from build123d import *

# Parameters (mm, degrees)
SKETCH_1_W          = 4.5
SKETCH_1_H          = 8
EXTRUDE_1_DEPTH     = 30
SKETCH_4_R          = 2.5
CUT_EXTRUDE_2_DEPTH = 32.372758884
SKETCH_7_R          = 3.5
CUT_EXTRUDE_4_DEPTH = 0.5
FILLET_1_R          = 1


with BuildPart() as part:
    # 草图1 → 凸台-拉伸1 (new body)
    with BuildSketch(Plane.XY):
        with Locations((2.25, 4)):
            Rectangle(SKETCH_1_W, SKETCH_1_H)
    extrude(amount=EXTRUDE_1_DEPTH)

    # 草图4 → 切除-拉伸2 (cut, through all)
    with BuildSketch(Plane(origin=(4.5, 0, 0), x_dir=(0, 0, -1), z_dir=(1, 0, 0))):
        with Locations((-5, 4)):
            Circle(SKETCH_4_R)
        with Locations((-22, 4)):
            Circle(SKETCH_4_R)
    extrude(amount=-CUT_EXTRUDE_2_DEPTH, mode=Mode.SUBTRACT)

    # 草图7 → 切除-拉伸4 (cut)
    with BuildSketch(Plane.ZY):
        with Locations((5, 4)):
            Circle(SKETCH_7_R)
        with Locations((22, 4)):
            Circle(SKETCH_7_R)
    extrude(amount=-CUT_EXTRUDE_4_DEPTH, mode=Mode.SUBTRACT)

    # 圆角1
    # the kernel refuses this fillet: 1 mm, written as the material it takes off along each edge
    with BuildSketch(Plane(origin=(3.5, 7, 29), x_dir=(1, 0, 0), z_dir=(0, 1, 0))) as fillet_1_piece_1_section:
        Polygon((0, 0), (FILLET_1_R, 0), (FILLET_1_R, -FILLET_1_R), (0, -FILLET_1_R), align=None)
    fillet_1_piece_1 = extrude(amount=FILLET_1_R, mode=Mode.PRIVATE)
    fillet_1_piece_1 = fillet_1_piece_1 - Plane(origin=(3.5, 7, 29), x_dir=(-0.7071067811865475, 0, -0.7071067811865475), z_dir=(0, 1, 0)) * Sphere(FILLET_1_R, mode=Mode.PRIVATE)
    add(fillet_1_piece_1, mode=Mode.SUBTRACT)
    with BuildSketch(Plane(origin=(3.5, 1, 29), x_dir=(0, 0, 1), z_dir=(1, 0, 0))) as fillet_1_piece_2_section:
        Polygon((0, 0), (FILLET_1_R, 0), (FILLET_1_R, FILLET_1_R), (0, FILLET_1_R), align=None)
    fillet_1_piece_2 = extrude(amount=FILLET_1_R, mode=Mode.PRIVATE)
    fillet_1_piece_2 = fillet_1_piece_2 - Plane(origin=(3.5, 1, 29), x_dir=(0, 0.7071067811865475, -0.7071067811865475), z_dir=(1, 0, 0)) * Sphere(FILLET_1_R, mode=Mode.PRIVATE)
    add(fillet_1_piece_2, mode=Mode.SUBTRACT)
    with BuildSketch(Plane(origin=(1, 7, 29), x_dir=(-1, 0, 0), z_dir=(0, 1, 0))) as fillet_1_piece_3_section:
        Polygon((0, 0), (FILLET_1_R, 0), (FILLET_1_R, FILLET_1_R), (0, FILLET_1_R), align=None)
    fillet_1_piece_3 = extrude(amount=FILLET_1_R, mode=Mode.PRIVATE)
    fillet_1_piece_3 = fillet_1_piece_3 - Plane(origin=(1, 7, 29), x_dir=(0.7071067811865475, 0, -0.7071067811865475), z_dir=(0, 1, 0)) * Sphere(FILLET_1_R, mode=Mode.PRIVATE)
    add(fillet_1_piece_3, mode=Mode.SUBTRACT)
    with BuildSketch(Plane(origin=(1, 1, 29), x_dir=(0, 0, 1), z_dir=(-1, 0, 0))) as fillet_1_piece_4_section:
        Polygon((0, 0), (FILLET_1_R, 0), (FILLET_1_R, -FILLET_1_R), (0, -FILLET_1_R), align=None)
    fillet_1_piece_4 = extrude(amount=FILLET_1_R, mode=Mode.PRIVATE)
    fillet_1_piece_4 = fillet_1_piece_4 - Plane(origin=(1, 1, 29), x_dir=(0, 0.7071067811865475, -0.7071067811865475), z_dir=(-1, 0, 0)) * Sphere(FILLET_1_R, mode=Mode.PRIVATE)
    add(fillet_1_piece_4, mode=Mode.SUBTRACT)
    with BuildSketch(Plane(origin=(1, 7, 1), x_dir=(-1, 0, 0), z_dir=(0, 1, 0))) as fillet_1_piece_5_section:
        Polygon((0, 0), (FILLET_1_R, 0), (FILLET_1_R, -FILLET_1_R), (0, -FILLET_1_R), align=None)
    fillet_1_piece_5 = extrude(amount=FILLET_1_R, mode=Mode.PRIVATE)
    fillet_1_piece_5 = fillet_1_piece_5 - Plane(origin=(1, 7, 1), x_dir=(0.7071067811865475, 0, 0.7071067811865475), z_dir=(0, 1, 0)) * Sphere(FILLET_1_R, mode=Mode.PRIVATE)
    add(fillet_1_piece_5, mode=Mode.SUBTRACT)
    with BuildSketch(Plane(origin=(3.5, 7, 1), x_dir=(1, 0, 0), z_dir=(0, 1, 0))) as fillet_1_piece_6_section:
        Polygon((0, 0), (FILLET_1_R, 0), (FILLET_1_R, FILLET_1_R), (0, FILLET_1_R), align=None)
    fillet_1_piece_6 = extrude(amount=FILLET_1_R, mode=Mode.PRIVATE)
    fillet_1_piece_6 = fillet_1_piece_6 - Plane(origin=(3.5, 7, 1), x_dir=(-0.7071067811865475, 0, 0.7071067811865475), z_dir=(0, 1, 0)) * Sphere(FILLET_1_R, mode=Mode.PRIVATE)
    add(fillet_1_piece_6, mode=Mode.SUBTRACT)
    with BuildSketch(Plane(origin=(3.5, 1, 1), x_dir=(0, 0, -1), z_dir=(1, 0, 0))) as fillet_1_piece_7_section:
        Polygon((0, 0), (FILLET_1_R, 0), (FILLET_1_R, -FILLET_1_R), (0, -FILLET_1_R), align=None)
    fillet_1_piece_7 = extrude(amount=FILLET_1_R, mode=Mode.PRIVATE)
    fillet_1_piece_7 = fillet_1_piece_7 - Plane(origin=(3.5, 1, 1), x_dir=(0, 0.7071067811865475, 0.7071067811865475), z_dir=(1, 0, 0)) * Sphere(FILLET_1_R, mode=Mode.PRIVATE)
    add(fillet_1_piece_7, mode=Mode.SUBTRACT)
    with BuildSketch(Plane(origin=(1, 1, 1), x_dir=(0, 0, -1), z_dir=(-1, 0, 0))) as fillet_1_piece_8_section:
        Polygon((0, 0), (FILLET_1_R, 0), (FILLET_1_R, FILLET_1_R), (0, FILLET_1_R), align=None)
    fillet_1_piece_8 = extrude(amount=FILLET_1_R, mode=Mode.PRIVATE)
    fillet_1_piece_8 = fillet_1_piece_8 - Plane(origin=(1, 1, 1), x_dir=(0, 0.7071067811865475, 0.7071067811865475), z_dir=(-1, 0, 0)) * Sphere(FILLET_1_R, mode=Mode.PRIVATE)
    add(fillet_1_piece_8, mode=Mode.SUBTRACT)
    with BuildSketch(Plane(origin=(4.5, 7, 30), x_dir=(0, 0, -1), z_dir=(0, -1, 0)), Plane(origin=(0, 1, 30), x_dir=(0, 0, -1), z_dir=(0, 1, 0))) as fillet_1_piece_9:
        with BuildLine():
            CenterArc((FILLET_1_R, -FILLET_1_R), FILLET_1_R, 90, 90)
            Line((0, -FILLET_1_R), (0, 0))
            Line((0, 0), (FILLET_1_R, 0))
        make_face()
    extrude(amount=6, mode=Mode.SUBTRACT)
    with BuildSketch(Plane(origin=(1, 8, 30), x_dir=(0, 0, -1), z_dir=(1, 0, 0)), Plane(origin=(3.5, 0, 0), x_dir=(0, 1, 0), z_dir=(-1, 0, 0))) as fillet_1_piece_10:
        with BuildLine():
            CenterArc((FILLET_1_R, -FILLET_1_R), FILLET_1_R, 90, 90)
            Line((0, -FILLET_1_R), (0, 0))
            Line((0, 0), (FILLET_1_R, 0))
        make_face()
    extrude(amount=2.5, mode=Mode.SUBTRACT)
    with BuildSketch(Plane(origin=(1, 8, 0), x_dir=(0, 0, 1), z_dir=(1, 0, 0)), Plane(origin=(3.5, 0, 30), x_dir=(0, 1, 0), z_dir=(-1, 0, 0))) as fillet_1_piece_11:
        with BuildLine():
            CenterArc((FILLET_1_R, FILLET_1_R), FILLET_1_R, 180, 90)
            Line((0, FILLET_1_R), (0, 0))
            Line((0, 0), (FILLET_1_R, 0))
        make_face()
    extrude(amount=2.5, mode=Mode.SUBTRACT)
    with BuildSketch(Plane(origin=(4.5, 7, 0), x_dir=(0, 0, 1), z_dir=(0, -1, 0)), Plane(origin=(0, 1, 0), x_dir=(0, 0, 1), z_dir=(0, 1, 0))) as fillet_1_piece_12:
        with BuildLine():
            CenterArc((FILLET_1_R, FILLET_1_R), FILLET_1_R, 180, 90)
            Line((0, FILLET_1_R), (0, 0))
            Line((0, 0), (FILLET_1_R, 0))
        make_face()
    extrude(amount=6, mode=Mode.SUBTRACT)
    with BuildSketch(Plane(origin=(0, 8, 1), x_dir=(1, 0, 0), z_dir=(0, 0, 1)), Plane(origin=(0, 0, 1), x_dir=(0, 1, 0), z_dir=(0, 0, 1))) as fillet_1_piece_13:
        with BuildLine():
            CenterArc((FILLET_1_R, -FILLET_1_R), FILLET_1_R, 90, 90)
            Line((0, -FILLET_1_R), (0, 0))
            Line((0, 0), (FILLET_1_R, 0))
        make_face()
    extrude(amount=28, mode=Mode.SUBTRACT)
    with BuildSketch(Plane(origin=(4.5, 8, 1), x_dir=(-1, 0, 0), z_dir=(0, 0, 1)), Plane(origin=(4.5, 0, 1), x_dir=(0, 1, 0), z_dir=(0, 0, 1))) as fillet_1_piece_14:
        with BuildLine():
            CenterArc((FILLET_1_R, FILLET_1_R), FILLET_1_R, 180, 90)
            Line((0, FILLET_1_R), (0, 0))
            Line((0, 0), (FILLET_1_R, 0))
        make_face()
    extrude(amount=28, mode=Mode.SUBTRACT)


solid = part.part
Design review of the part built by this model. Coordinates are the model's own, in mm. A direction names the side the tool comes from. Round coordinates to 2 decimals unless told otherwise and drop trailing zeros. Loops run counter-clockwise (first coordinate to the right, second up) from the corner with the lowest first, then second, coordinate; pieces in that order, holes last. Notation, with made-up numbers: (-16.75, 33) - (1.25, 33) arc R22 ccw to (1.25, 72) - close; hole circle Ø4 at (46, -6.5). An arc over 180 degrees is marked (long way). One line per question, with ' | ' between items.
1. Clearance check with a flat-ended pin moving along its axis: P1, Ø3.5, axis at y = 2.5, z = 5, coming from the -X side. State where the tip first meets the part, or that it passes through.
Results are:
P1: stops at x = 0.5
2. For L1, parallel to Y at x = 2.05, z = 22; L2, parallel to Z at x = 0.3, y = 4; L3, parallel to Z at x = 0.2, y = 4, list the stretches that pass through material, from the lowest coordinate up. Write a range as [from, to].
Results are:
L1: y = [0, 1.5], [6.5, 8] | L2: z = [0.29, 1.5], [8.5, 18.5], [25.5, 29.71] | L3: z = [0.4, 1.5], [8.5, 18.5], [25.5, 29.6]
3. Draft analysis for pull direction Z (two halves, no side actions). For faces 3 (the face through (2.5, 4.1, 24.5)), 4 (the face through (2.232, 7.715, 29.699)), 5 (the face through (4.5, 4, 15)), state which applies: released by +Z, released by -Z, zero draft, split by the parting line, or undercut.
Results are:
face 3: undercut | face 4: released by +Z | face 5: zero draft
4. We need section B-B, the plane x = 2.3. State the section outline as (y, z) points, and give its area (3 significant figures).
Results are:
outline: (0, 1) arc R1 ccw to (1, 0) - (7, 0) arc R1 ccw to (8, 1) - (8, 29) arc R1 ccw to (7, 30) - (1, 30) arc R1 ccw to (0, 29) - close; hole circle Ø5 at (4, 5); hole circle Ø5 at (4, 22) | area: 200 mm²
5. For faces 1 (the face through (2.268, 0.301, 0.285)), 2 (the face through (0.246, 2.659, 8.233)), list the 3-axis set-ups (+Z, -Z, +X, -X, +Y, -Y) from which the entire face can be reached by the end or side of a thin tool; tool diameter is ignored.
Results are:
face 1: -Z, +X, -X, -Y | face 2: -X
6. We need section A-A, the plane y = 4. State the section outline as (x, z) points, and give its area (3 significant figures).
Results are:
outline: (0, 1) arc R1 ccw to (1, 0) - (3.5, 0) arc R1 ccw to (4.5, 1) - (4.5, 2.5) - (0.5, 2.5) - (0.5, 1.5) - (0, 1.5) - close; (0, 8.5) - (0.5, 8.5) - (0.5, 7.5) - (4.5, 7.5) - (4.5, 19.5) - (0.5, 19.5) - (0.5, 18.5) - (0, 18.5) - close; (0, 25.5) - (0.5, 25.5) - (0.5, 24.5) - (4.5, 24.5) - (4.5, 29) arc R1 ccw to (3.5, 30) - (1, 30) arc R1 ccw to (0, 29) - close | area: 87.1 mm²
7. We need section C-C, the plane z = 5. State the section outline as (x, y) points, and give its area (3 significant figures).
Results are:
outline: (0.13, 0.5) arc R1 ccw to (1, 0) - (3.5, 0) arc R1 ccw to (4.5, 1) - (4.5, 1.5) - (0.5, 1.5) - (0.5, 0.5) - close; (0.13, 7.5) - (0.5, 7.5) - (0.5, 6.5) - (4.5, 6.5) - (4.5, 7) arc R1 ccw to (3.5, 8) - (1, 8) arc R1 ccw to start | area: 11.7 mm²
